```python
from build123d import *

# Parameters (mm, degrees)
F0_R      = 18.034
F1_DEPTH  = 57.2516
F2_R      = 6.477
F3_DEPTH  = 4.3434
F4_R      = 1.27
F5_R      = 4.826
F6_DEPTH  = 0.508
F7_R      = 1.5875
F8_DEPTH  = 19.177
F9_W      = 18.161
F9_H      = 1.016
F10_DEPTH = 3.175
F11_R     = 17.3228
F12_DEPTH = 1.27
F13_W     = 3.81
F13_H     = 0.508
F14_DEPTH = 7.874
F16_SIZE  = 0.889
F17_R     = 1.27
F18_W     = 0.2921
F18_H     = 1.524
F18_W_2   = 1.905
F18_H_2   = 2.413
F19_DEPTH = 29.0957


with BuildPart() as f1:
    # F0 (on Front) → F1 (new body)
    with BuildSketch(Plane.XZ):
        Circle(F0_R)
    extrude(amount=F1_DEPTH)

    # F2 (on face) → F3 (join)
    with BuildSketch(Plane.XZ.offset(57.2516)):
        Circle(F2_R)
    extrude(amount=F3_DEPTH)

    # F4
    f4_edges = [f1.edges().sort_by_distance(p)[0] for p in [
        (-6.477, -57.2516, 0),
        (-6.477, -61.595, 0),
    ]]
    fillet(f4_edges, radius=F4_R)

    # F5 (on face) → F6 (cut)
    with BuildSketch(Plane.XZ.offset(61.595)):
        Circle(F5_R)
    extrude(amount=-F6_DEPTH, mode=Mode.SUBTRACT)

    # F7 (on face) → F8 (join)
    with BuildSketch(Plane.XZ.offset(61.087)):
        Circle(F7_R)
    extrude(amount=F8_DEPTH)

    # F9 (on Right) → F10 (cut, symmetric)
    with BuildSketch(Plane.YZ):
        with Locations((-71.1835, 1.0795)):
            Rectangle(F9_W, F9_H)
    extrude(amount=F10_DEPTH, both=True, mode=Mode.SUBTRACT)

    # F11 (on face) → F12 (cut)
    with BuildSketch(Plane(origin=(0, 0, 0), x_dir=(-1, 0, 0), z_dir=(0, 1, 0))):
        Circle(F11_R)
    extrude(amount=-F12_DEPTH, mode=Mode.SUBTRACT)

    # F13 (on face) → F14 (join)
    with BuildSketch(Plane(origin=(0, -1.27, 0), x_dir=(-1, 0, 0), z_dir=(0, 1, 0))):
        with Locations((0, 14.2748)):
            Rectangle(F13_W, F13_H)
        with Locations((0, -14.2748)):
            Rectangle(F13_W, F13_H)
    extrude(amount=F14_DEPTH)

    # F16
    f16_edges = [f1.edges().sort_by_distance(p)[0] for p in [
        (-1.905, 6.604, 14.2748),
        (1.905, 6.604, 14.2748),
        (-1.905, 6.604, -14.2748),
        (1.905, 6.604, -14.2748),
    ]]
    chamfer(f16_edges, length=F16_SIZE)

    # F17
    f17_edges = [f1.edges().sort_by_distance(p)[0] for p in [
        (-18.034, -57.2516, 0),
    ]]
    fillet(f17_edges, radius=F17_R)

    # F18 (on face) → F19 (cut)
    with BuildSketch(Plane.XY.offset(14.5288)):
        with Locations((-1.75895, -0.508)):
            Rectangle(F18_W, F18_H)
        with Locations((1.75895, -0.508)):
            Rectangle(F18_W, F18_H)
        with Locations((0, 3.7719)):
            Rectangle(F18_W_2, F18_H_2)
    extrude(amount=-F19_DEPTH, mode=Mode.SUBTRACT)


solid = f1.part
```
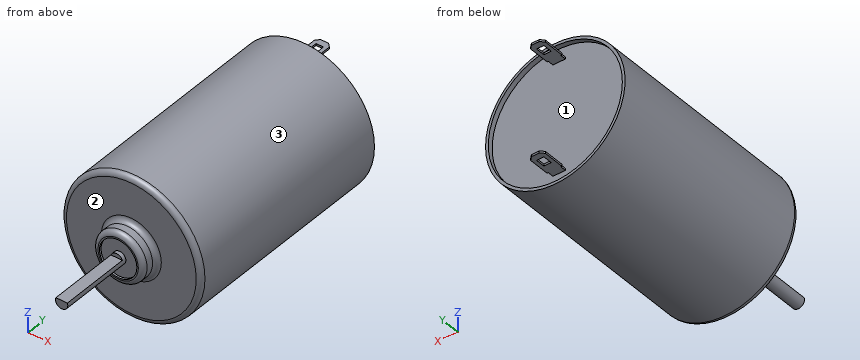
Here's how the part is built. I have some questions about the finished solid (model axes, mm). Face numbers are marked on the shaded views. Coordinates: 2 decimals unless noted, no trailing zeros. Loops run counter-clockwise (first coordinate to the right, second up) from the corner with the lowest first, then second, coordinate; pieces in that order, holes last. Notation, with made-up numbers: M 57,-23 L 69,-23 A25 cw 69,4 Z; hole C 68.5,-25 d3. An arc over 180 degrees is marked long. One line per item, written item: value.
1. Imagine slicing it at B-B (y = -30.5). List the corners of the cut face in (x, z) for me.
Geometry says:
outline: C 0,0 d36.07
2. Imagine slicing it at A-A (x = 0). State how many separate pieces and enclosed holes the cut face has, and give its area (3 significant figures).
Geometry says:
separate pieces: 3
enclosed holes: 0
area: 2,120 mm2
3. Thinking about a two-plate mould opening in X: for the marked faces 1, 2 and 3, which applies, +X half, -X half, draft (parallel to the pull), parting line (faces both ways), or undercut?
Geometry says:
face 1: undercut
face 2: draft
face 3: parting line
4. Please list where these lines run through material, in increasing order: probe 1 along Z at (x, y) = (0, -61.4); probe 2 along Y at (x, z) = (-8.5, -5); probe 3 along Y at (x, z) = (1, 0).
Geometry says:
probe 1: z = -5.88 to -4.83, -1.59 to 1.59, 4.83 to 5.88
probe 2: y = -57.25 to -1.27
probe 3: y = -80.26 to -1.27
5. Will these pins go through, and if not, where does the flat tip stop? pin 1 Ø10 at (x, y) = (6.5, -12) entering from -Z; pin 2 Ø11 at (x, z) = (0, 0) entering from +Y; pin 3 Ø1.1 at (x, y) = (-0.5, 3) entering from +Z.
Geometry says:
pin 1: stops at z = -17.97
pin 2: stops at y = -1.27
pin 3: stops at z = 14.53
